Source: CAD feature listing. Evaluate the final solid. Frame: model axes, mm. Round coordinates to 2 decimals unless told otherwise and drop trailing zeros. Loops run counter-clockwise (first coordinate to the right, second up) from the corner with the lowest first, then second, coordinate; pieces in that order, holes last. Notation, with made-up numbers: M 4.25,-21.5 L 48.25,-21.5 A21 ccw 48.25,-5.5 Z; hole C 23.5,8 d5. An arc over 180 degrees is marked long. Answer as CSV lines item,"result". Start each with the question number.
```python
from build123d import *

# Parameters (mm, degrees)
F1_DEPTH = 37.846
F2_R     = 7.4693971268
F3_DEPTH = 80.2441237786
F4_R     = 7.1391458969
F5_DEPTH = 37.847
F6_R     = 6.8840617495
F7_DEPTH = 80.2441237786
F8_R     = 9.6297626658
F9_DEPTH = 37.847


with BuildPart() as f1:
    # F0 (on Top) → F1 (new body)
    with BuildSketch(Plane.XY):
        Polygon((-67.0226588845, 34.8154716194), (-66.8756216764, -48.5164038837), (17.8625807166, -24.6178079396), align=None)
    extrude(amount=F1_DEPTH)

    # F2 (on face) → F3 (cut, through all)
    with BuildSketch(Plane(origin=(7.7474819604, -27.4705550039, 0), x_dir=(0.9624553813, 0.2714399364, 0), z_dir=(0.2714399364, -0.9624553813, 0))):
        with Locations((-54.2420856655, 21.0362523794)):
            Circle(F2_R)
    extrude(amount=-F3_DEPTH, mode=Mode.SUBTRACT)

    # F4 (on face) → F5 (cut, through all)
    with BuildSketch(Plane.XY.offset(37.846)):
        with Locations((-13.3007261902, -23.1652185321)):
            Circle(F4_R)
    extrude(amount=-F5_DEPTH, mode=Mode.SUBTRACT)

    # F6 (on face) → F7 (cut, through all)
    with BuildSketch(Plane(origin=(7.7474819604, -27.4705550039, 0), x_dir=(0.9624553813, 0.2714399364, 0), z_dir=(0.2714399364, -0.9624553813, 0))):
        with Locations((-4.4350521639, 11.9895972311)):
            Circle(F6_R)
    extrude(amount=-F7_DEPTH, mode=Mode.SUBTRACT)

    # F8 (on face) → F9 (cut, through all)
    with BuildSketch(Plane.XY.offset(37.846)):
        with Locations((-52.3273982108, 0)):
            Circle(F8_R)
    extrude(amount=-F9_DEPTH, mode=Mode.SUBTRACT)


solid = f1.part
```
1) Contact query for flat-ended pins moving along their axis: pin 1 Ø1.5 at (x, z) = (-32.5, 10) entering from +Y; pin 2 Ø6 at (y, z) = (-9.5, 15) entering from -X; pin 3 Ø1.5 at (x, z) = (-12.5, 5.5) entering from +Y. Output: stop coordinate, or through.
2) Section D-D, the plane x = -32. Return loops of the section in (y, z).
3) Mould query, pull axis X, two halves, no side actions, for faces 1 (the cylindrical face through (-5.946, -20.594, 12.292)), 2 (the flat face through (-35, -16, 0)), 3 (the flat face through (-23.986, 4.683, 18.658)). Classes: pulls with the +X half, pulls with the -X half, needs draft (parallel to the pull), parting line crosses it, or undercut.
4) Section A-A, the plane z = 7. Return loops of the section in (x, y).
5) Section B-B, the plane y = -20. Give the number of separate pieces and of enclosed holes in the cut face, and give its area (3 significant figures).
6) Ray query, line 1 along X through (y, z) = (-17.5, 7) (3 decimals); line 2 along Y through (x, z) = (-16, 22); line 3 along X through (y, z) = (-8, 14). Return the intervals inside material, ascending.
7) Section C-C, the plane z = 30. Return loops of the section in (x, y).
Findings below:
1,pin 1,"y = 11.17"
1,pin 2,"x = -66.95"
1,pin 3,"y = -2.83"
2,outline,"M -38.68,0 L 10.29,0 L 10.29,37.85 L -38.68,37.85 Z"
3,face 1,"undercut"
3,face 2,"needs draft"
3,face 3,"pulls with the +X half"
4,outline,"M -67.02,34.82 L -66.88,-48.52 L -1.09,-29.96 L -7.63,-6.77 Z; M 4.65,-15.37 L 8.04,-27.39 L 17.86,-24.62 Z; hole C -52.33,0 d19.26; hole C -13.3,-23.17 d14.28"
5,separate pieces,"2"
5,enclosed holes,"2"
5,area,"2,140 mm²"
6,line 1,"-66.93 to -17.645, -8.956 to -4.6, 5.255 to 7.697"
6,line 2,"-34.17 to -29.77, -16.56 to -0.91"
6,line 3,"-66.95 to -57.69, -46.97 to -9.19"
7,outline,"M -67.02,34.82 L -66.88,-48.52 L 17.86,-24.62 Z; hole C -52.33,0 d19.26; hole C -13.3,-23.17 d14.28"
